Input: part model. Units: mm. Frame: model coordinates. Coordinates: 2 decimals unless noted, no trailing zeros. Order: outer loops, then holes, each group sorted by start corner. A loop starts at its lowest first (then second) coordinate and runs counter-clockwise, first axis right, second up. Notation, with made-up numbers: (54, -4.75) -> (73, -4.75) arc R30 ccw to (73, 33.25) -> close; hole circle Ø4 at (79, 79). An arc over 180 degrees is marked (long way). Use CSV: the item, a comma, the result in double quotes. Start each with the question number.
```python
from build123d import *

# Parameters (mm, degrees)
BOSS_EXTRUDE1_DEPTH = 3
SKETCH2_R           = 3
BOSS_EXTRUDE2_DEPTH = 6


with BuildPart() as part:
    # Sketch1 → Boss-Extrude1 (new body)
    with BuildSketch(Plane.XY):
        with BuildLine():
            Line((250, 382.208907076), (-250, 382.208907076))
            add(Edge.make_bspline(
                [(-250, 382.208907076), (-260.435607626, 382.208907076), (-270, 376.305635941)],
                knots=[0, 0, 0, 0.411516846, 0.411516846, 0.411516846], degree=2, weights=[1, 0.978906313, 1]))
            Line((-270, 376.305635941), (-270, 624.340941432))
            add(Edge.make_bspline(
                [(-250, 652.625212679), (-270, 652.625212679), (-270, 624.340941432)],
                knots=[0, 0, 0, 1.570796327, 1.570796327, 1.570796327], degree=2, weights=[1, 0.707106781, 1]))
            Line((-250, 652.625212679), (250, 652.625212679))
            add(Edge.make_bspline(
                [(270, 624.340941432), (270, 652.625212679), (250, 652.625212679)],
                knots=[1.570796327, 1.570796327, 1.570796327, 3.141592654, 3.141592654, 3.141592654], degree=2, weights=[1, 0.707106781, 1]))
            Line((270, 624.340941432), (270, 376.305635941))
            add(Edge.make_bspline(
                [(270, 376.305635941), (260.435607626, 382.208907076), (250, 382.208907076)],
                knots=[2.730075808, 2.730075808, 2.730075808, 3.141592654, 3.141592654, 3.141592654], degree=2, weights=[1, 0.978906313, 1]))
        make_face()
    extrude(amount=-BOSS_EXTRUDE1_DEPTH)

    # Sketch2 → Boss-Extrude2 (add)
    with BuildSketch(Plane.XY):
        with Locations((-30, 392.208907076)):
            Circle(SKETCH2_R)
        with Locations((210, 392.208907076)):
            Circle(SKETCH2_R)
    extrude(amount=BOSS_EXTRUDE2_DEPTH)


solid = part.part
```
1. Material intervals for line 1 along Z through (x, y) = (-163, 558); line 2 along Y through (x, z) = (114, -1.5), sorted ascending.
2. Contact query for flat-ended pins moving along their axis: P1, Ø2.5, axis at x = 61, z = -2, coming from the -Y side; P2, Ø5, axis at x = -132, y = 521, coming from the +Z side. Output: stop coordinate, or through.
3. Section C-C on z = 2.75. Return loops of the section in (x, y), then the cut area to 3 significant figures.
4. Section A-A on x = -85. Return loops of the section in (y, z).
5. Section B-B on y = 405. Return loops of the section in (x, z), then the cut area to 3 significant figures.
Values follow:
1,line 1,"z = -3 to 0"
1,line 2,"y = 382.21 to 652.63"
2,P1,"stops at y = 382.21"
2,P2,"stops at z = 0"
3,outline,"circle Ø6 at (-30, 392.21); circle Ø6 at (210, 392.21)"
3,area,"56.5 mm2"
4,outline,"(382.21, -3) -> (652.63, -3) -> (652.63, 0) -> (382.21, 0) -> close"
5,outline,"(-270, -3) -> (270, -3) -> (270, 0) -> (-270, 0) -> close"
5,area,"1,620 mm2"
